Can you work these out from the model? Positions are in its coordinate system, mm. Face numbers are marked on the shaded views. Give positions to 0.01 mm unless a question says otherwise; leave off trailing zeros. Write each loop counter-clockwise with the first axis right and the second up, starting at its lowest first coordinate (ties: lowest second). Pieces come first, ordered by that corner, then holes.
1. Suppose I cut it at A-A (y = 4.75). Please give me the cut outline in (x, z), and give its area (3 significant figures).
2. Thinking about a two-plate mould opening in X: for the marked faces 1 and 2, which applies, pulls with the +X half, pulls with the -X half, needs draft (parallel to the pull), parting line crosses it, or undercut?
3. If I drill on probe 1 along X at (y, z) = (5.5, -643); probe 2 along X at (y, z) = (0.75, 202); probe 3 along Y at (x, z) = (-55, 294), over which ranges is the centre line in solid material (lowest first)?
4. Suppose I cut it at B-B (z = 712). Please give me the cut outline in (x, y).
5. I'm going to push a flat-ended pin straight in: pin 1 (8 mm diameter, centred on x = 83, z = -634, fed in from +Y). Where does the tip first touch, or does it pass through?
6. Suppose I cut it at C-C (x = -139.5). Please give me the cut outline in (y, z).
Autodesk Inventor part; units mm, degrees
ref_plane "YZ Plane" through (0, 0, 0) normal (1, 0, 0) x (0, 1, 0)
ref_plane "XZ Plane" through (0, 0, 0) normal (0, 1, 0) x (-1, 0, 0)
ref_plane "XY Plane" through (0, 0, 0) normal (0, 0, 1) x (1, 0, 0)
sketch "Sketch6" plane through (0, 0, 0) normal (0, 1, 0) x (-1, 0, 0)
  line L0 (205.5, -990) -> (-205.5, -990)
  line L1 (-205.5, -990) -> (-205.5, 990)
  line L2 (-205.5, 990) -> (205.5, 990)
  line L3 (205.5, 990) -> (205.5, -990)
  line L4 (205.5, -990) -> (-205.5, 990) construction
  line L5 (-205.5, -990) -> (205.5, 990) construction
  point P0 (0, 0)
  dimension "d52" = 411
  dimension "d53" = 1980
extrude "Plate2" add sketch "Sketch6" along normal blind 0.5
sketch "Sketch12" plane through (-205, 0, 990) normal (-1, 0, 0) x (0, -1, 0)
  line L0 (0, -1980) -> (0, 0)
  line L1 (0, 0) -> (-10, 0)
  line L2 (-10, 0) -> (-10, -1980)
  line L3 (-10, -1980) -> (0, -1980)
edge flange "Flange3" height 10 angle 90 thickness 0.5 bend radius 0.5 thickness toward (-1, 0, 0) relief tear relief width 0.5 relief depth 0.25 edges at (-205.5, 0.5, 0) wall of the first edge with corners at (-205, 0, -990) (-205, 0, 990) (-205, 10, 990) (-205, 10, -990)
bend "Bend4"
corner "Corner4"
sketch "Sketch13" plane through (-205.5, 9.5, 990) normal (0, 1, 0) x (-1, 0, 0)
  line L0 (0, -1980) -> (0, 0)
  line L1 (0, 0) -> (-10, 0)
  line L2 (-10, 0) -> (-10, -1980)
  line L3 (-10, -1980) -> (0, -1980)
edge flange "Flange4" height 10 angle 90 thickness 0.5 bend radius 0.5 thickness toward (0, 1, 0) relief tear relief width 0.5 relief depth 0.25 edges at (-205, 10, 0) wall of the first edge with corners at (-205.5, 9.5, -990) (-205.5, 9.5, 990) (-195.5, 9.5, 990) (-195.5, 9.5, -990)
bend "Bend5"
corner "Corner5"
sketch "Sketch14" plane through (205, 0, -990) normal (1, 0, 0) x (0, 1, 0)
  line L0 (0, 1980) -> (0, 0)
  line L1 (0, 0) -> (10, 0)
  line L2 (10, 0) -> (10, 1980)
  line L3 (10, 1980) -> (0, 1980)
edge flange "Flange5" height 10 angle 90 thickness 0.5 bend radius 0.5 thickness toward (1, 0, 0) relief tear relief width 0.5 relief depth 0.25 edges at (205.5, 0.5, 0) wall of the first edge with corners at (205, 0, 990) (205, 0, -990) (205, 10, -990) (205, 10, 990)
bend "Bend6"
corner "Corner6"
sketch "Sketch15" plane through (205.5, 9.5, -990) normal (0, 1, 0) x (-1, 0, 0)
  line L0 (0, 1980) -> (0, 0)
  line L1 (0, 0) -> (10, 0)
  line L2 (10, 0) -> (10, 1980)
  line L3 (10, 1980) -> (0, 1980)
edge flange "Flange6" height 10 angle 90 thickness 0.5 bend radius 0.5 thickness toward (0, 1, 0) relief tear relief width 0.5 relief depth 0.25 edges at (205, 10, 0) wall of the first edge with corners at (205.5, 9.5, 990) (205.5, 9.5, -990) (195.5, 9.5, -990) (195.5, 9.5, 990)
bend "Bend7"
corner "Corner7"
equation "\"d52\" = ЖАБРЫ_базовая_ширина - 5 * ЖАБРЫ_шаг_листов"
equation "\"d53\" = ЖАБРЫ_базовая_длина_дл_лист"
equation "\"d54\" = Thickness"
equation "\"d94\" = BendReliefWidth"
equation "\"d95\" = BendReliefDepth"
equation "\"d96\" = MinimumRemnant"
equation "\"d97\" = TransitionRadius"
equation "\"d100\" = BendRadius"
equation "\"d101\" = CornerReliefSize"
equation "\"d102\" = GapSize"
equation "\"d103\" = JacobiRadiusSize"
equation "\"d104\" = BendReliefWidth"
equation "\"d105\" = BendReliefDepth"
equation "\"d106\" = MinimumRemnant"
equation "\"d107\" = TransitionRadius"
equation "\"d110\" = BendRadius"
equation "\"d111\" = CornerReliefSize"
equation "\"d112\" = GapSize"
equation "\"d113\" = JacobiRadiusSize"
equation "\"d114\" = BendReliefWidth"
equation "\"d115\" = BendReliefDepth"
equation "\"d116\" = MinimumRemnant"
equation "\"d117\" = TransitionRadius"
equation "\"d120\" = BendRadius"
equation "\"d121\" = CornerReliefSize"
equation "\"d122\" = GapSize"
equation "\"d123\" = JacobiRadiusSize"
equation "\"d124\" = BendReliefWidth"
equation "\"d125\" = BendReliefDepth"
equation "\"d126\" = MinimumRemnant"
equation "\"d127\" = TransitionRadius"
equation "\"d130\" = BendRadius"
equation "\"d131\" = CornerReliefSize"
equation "\"d132\" = GapSize"
equation "\"d133\" = JacobiRadiusSize"
equation "\"BendRadius\" = Thickness"
equation "\"BendReliefWidth\" = Thickness"
equation "\"BendReliefDepth\" = 0.5 * Thickness"
equation "\"CornerReliefSize\" = 4 * Thickness"
equation "\"MinimumRemnant\" = 2 * Thickness"
equation "\"TransitionRadius\" = BendRadius"
equation "\"JacobiRadiusSize\" = BendRadius"
equation "\"GapSize\" = Thickness"
properties part number "MSC 812 sheet gills" material "Stainless Steel"
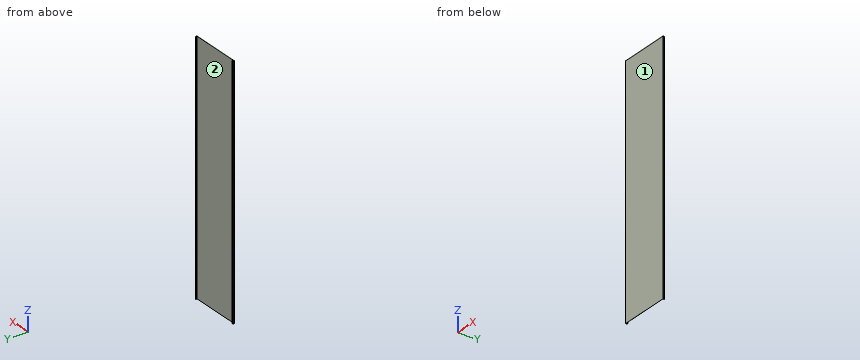
Checks:
1. outline: (-205.5, -990) - (-205, -990) - (-205, 990) - (-205.5, 990) - close; (205, -990) - (205.5, -990) - (205.5, 990) - (205, 990) - close
1. area: 1,980 mm2
2. face 1: needs draft
2. face 2: undercut
3. probe 1: x = -205.5 to -205, 205 to 205.5
3. probe 2: x = -205.47 to -204.93, 204.93 to 205.47
3. probe 3: y = 0 to 0.5
4. outline: (-205.5, 1) arc R1 ccw to (-204.5, 0) - (204.5, 0) arc R1 ccw to (205.5, 1) - (205.5, 9) arc R1 ccw to (204.5, 10) - (195.5, 10) - (195.5, 9.5) - (204.5, 9.5) arc R0.5 cw to (205, 9) - (205, 1) arc R0.5 cw to (204.5, 0.5) - (-204.5, 0.5) arc R0.5 cw to (-205, 1) - (-205, 9) arc R0.5 cw to (-204.5, 9.5) - (-195.5, 9.5) - (-195.5, 10) - (-204.5, 10) arc R1 ccw to (-205.5, 9) - close
5. pin 1: stops at y = 0.5
6. outline: (0, -990) - (0.5, -990) - (0.5, 990) - (0, 990) - close
